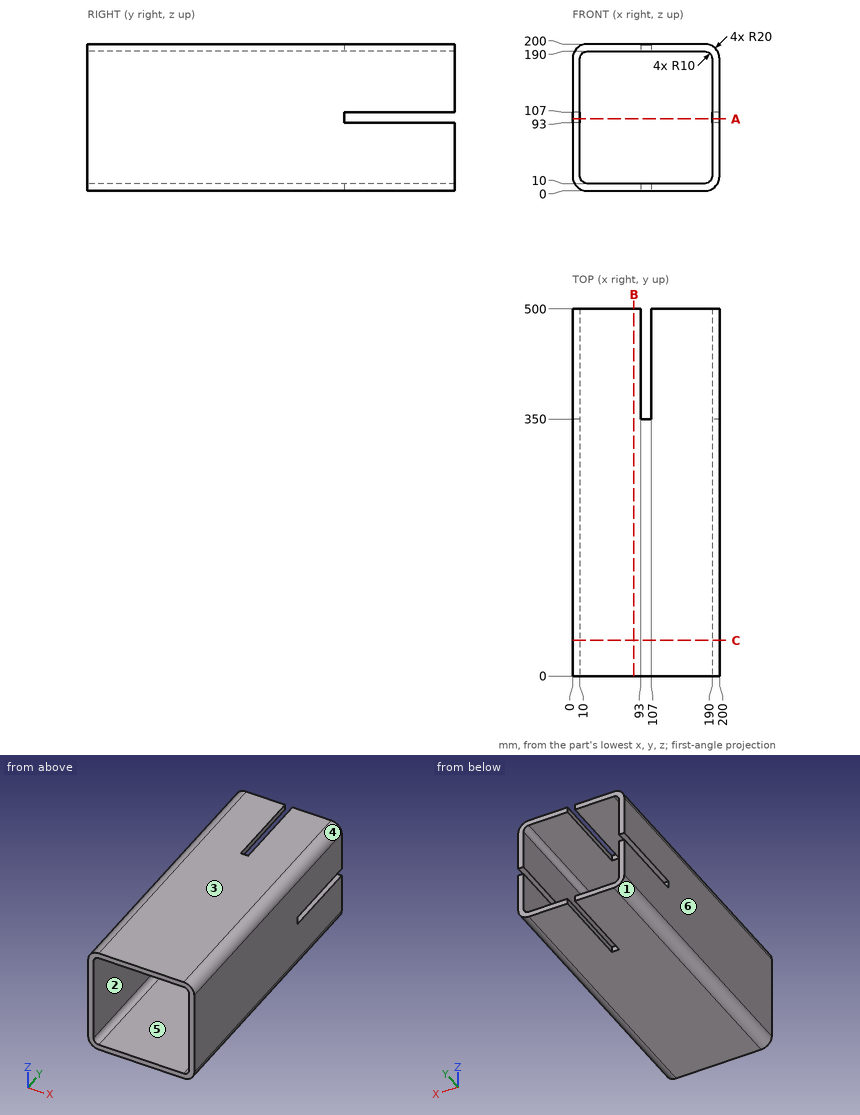
Here's the drawing with two shaded views (mm, measured from the low corner). I have some questions. A direction names the side the tool comes from. Coordinates: 2 decimals unless noted, no trailing zeros. Loops run counter-clockwise (first coordinate to the right, second up) from the corner with the lowest first, then second, coordinate; pieces in that order, holes last. Notation, with made-up numbers: (61.25, 43) -> (90.25, 43) arc R14 cw to (90.25, 57) -> close; hole circle Ø10 at (67, -26). An arc over 180 degrees is marked (long way). Answer in a Markdown table with one row per item.
(1) For the marked faces 1 and 2, which set-ups out of +Z, -Z, +X, -X, +Y, -Y let a thin tool reach every point of the face, with its end or its side?
Results found:
| item | result |
|---|---|
| face 1 | -Z, -X, +Y, -Y |
| face 2 | +Y, -Y |
(2) Imagine slicing it at B-B (x = 83.5). List the corners of the cut face in (y, z) for me.
Results found:
| item | result |
|---|---|
| outline | (0, 0) -> (500, 0) -> (500, 10) -> (0, 10) -> close; (0, 190) -> (500, 190) -> (500, 200) -> (0, 200) -> close |
(3) Imagine slicing it at A-A (z = 98). List the corners of the cut face in (x, y) for me, plus the area to 3 significant figures.
Results found:
| item | result |
|---|---|
| outline | (0, 0) -> (10, 0) -> (10, 350) -> (0, 350) -> close; (190, 0) -> (200, 0) -> (200, 350) -> (190, 350) -> close |
| area | 7,000 mm^2 |
(4) Imagine slicing it at C-C (y = 48.5). List the corners of the cut face in (x, z) for me.
Results found:
| item | result |
|---|---|
| outline | (0, 20) arc R20 ccw to (20, 0) -> (180, 0) arc R20 ccw to (200, 20) -> (200, 180) arc R20 ccw to (180, 200) -> (20, 200) arc R20 ccw to (0, 180) -> close; hole (10, 20) arc R10 ccw to (20, 10) -> (180, 10) arc R10 ccw to (190, 20) -> (190, 180) arc R10 ccw to (180, 190) -> (20, 190) arc R10 ccw to (10, 180) -> close |
(5) Will these pins go through, and if not, where does the flat tip stop? pin 1 Ø8 at (y, z) = (455, 5.5) entering from +X; pin 2 Ø5 at (x, y) = (6, 427.5) entering from -Z; pin 3 Ø5 at (x, y) = (5.5, 434) entering from +Z.
Results found:
| item | result |
|---|---|
| pin 1 | stops at x = 197.02 |
| pin 2 | stops at z = 3.64 |
| pin 3 | stops at z = 196 |
(6) If I drill on probe 1 along Z at (x, y) = (58, 321.5); probe 2 along Z at (x, y) = (187, 305.5) (3 decimals), over which ranges is the centre line in solid material (lowest first)?
Results found:
| item | result |
|---|---|
| probe 1 | z = 0 to 10, 190 to 200 |
| probe 2 | z = 1.265 to 12.859, 187.141 to 198.735 |
(7) Thinking about a two-plate mould opening in X: for the marked faces 3, 4, 5 and 6, which applies, released by +X, released by -X, zero draft, split by the parting line, or undercut?
Results found:
| item | result |
|---|---|
| face 3 | zero draft |
| face 4 | released by +X |
| face 5 | undercut |
| face 6 | released by -X |
